Source: CAD feature listing. Evaluate the final solid. Frame: model axes, mm. Give positions to 0.01 mm unless a question says otherwise; leave off trailing zeros. Order: outer loops, then holes, each group sorted by start corner. A loop starts at its lowest first (then second) coordinate and runs counter-clockwise, first axis right, second up. Notation, with made-up numbers: M -7,-32.5 L 25,-32.5 A18 ccw 25,-8.5 Z; hole C -30,4.25 d1. An arc over 180 degrees is marked long. Use CSV: the item, a comma, the result in double quotes. Start each with the question number.
1. Line query: line 1 along Y through (x, z) = (-74, 1.45); line 2 along Y through (x, z) = (-49.5, 0.8); line 3 along X through (y, z) = (42, 2.15). Output: solid intervals per line, ascending. Write a range as [from, to].
2. Section query B-B, the plane y = 65. Return the cut outline in (x, z), plus the area to 3 significant figures.
3. Section query A-A, the plane x = -74. Return the cut outline in (y, z), plus the area to 3 significant figures.
4. Section query C-C, the plane z = 1.8. Return the cut outline in (x, y), plus the area to 3 significant figures.
from build123d import *

# Parameters (mm, degrees)
ESQUISSE1_W             = 152
ESQUISSE1_H             = 165
BOSS_EXTRU_1_DEPTH      = 3
CONG_1_R                = 5
ESQUISSE2_R             = 47.5
ENL_V_MAT_EXTRU_1_DEPTH = 3
ENL_V_MAT_EXTRU_2_DEPTH = 3


with BuildPart() as part:
    # Esquisse1 → Boss.-Extru.1 (new body)
    with BuildSketch(Plane.XY):
        with Locations((-76, 82.5)):
            Rectangle(ESQUISSE1_W, ESQUISSE1_H)
    extrude(amount=BOSS_EXTRU_1_DEPTH)

    # Congé1
    cong_1_edges = [part.edges().sort_by_distance(p)[0] for p in [
        (0, 0, 1.5),
        (-152, 0, 1.5),
        (-152, 165, 1.5),
        (0, 165, 1.5),
    ]]
    fillet(cong_1_edges, radius=CONG_1_R)

    # Esquisse2 → Enlèv. mat.-Extru.1 (cut)
    with BuildSketch(Plane(origin=(0, 0, 0), x_dir=(-1, 0, 0), z_dir=(0, 0, -1))):
        with Locations((74, 65)):
            Circle(ESQUISSE2_R)
    extrude(amount=-ENL_V_MAT_EXTRU_1_DEPTH, mode=Mode.SUBTRACT)

    # Esquisse3 → Enlèv. mat.-Extru.2 (cut)
    with BuildSketch(Plane(origin=(0, 0, 0), x_dir=(-1, 0, 0), z_dir=(0, 0, -1))):
        with BuildLine():
            Line((37, -3), (37, 3))
            ThreePointArc((37, 3), (41, 7), (45, 3))
            Line((45, 3), (45, -3))
            ThreePointArc((45, -3), (41, -7), (37, -3))
        make_face()
        with BuildLine():
            Line((103, -3), (103, 3))
            ThreePointArc((103, 3), (107, 7), (111, 3))
            Line((111, 3), (111, -3))
            ThreePointArc((111, -3), (107, -7), (103, -3))
        make_face()
    extrude(amount=-ENL_V_MAT_EXTRU_2_DEPTH, mode=Mode.SUBTRACT)


solid = part.part
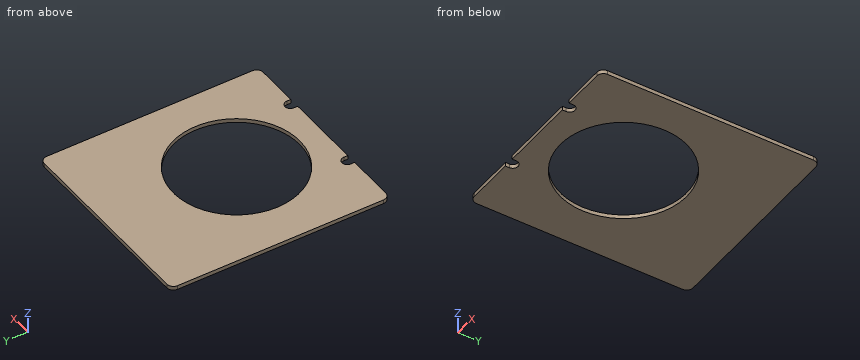
Result set:
1,line 1,"[0, 17.5], [112.5, 165]"
1,line 2,"[0, 24.31], [105.69, 165]"
1,line 3,"[-152, -115.56], [-32.44, 0]"
2,outline,"M -152,0 L -121.5,0 L -121.5,3 L -152,3 Z; M -26.5,0 L 0,0 L 0,3 L -26.5,3 Z"
2,area,"171 mm2"
3,outline,"M 0,0 L 17.5,0 L 17.5,3 L 0,3 Z; M 112.5,0 L 165,0 L 165,3 L 112.5,3 Z"
3,area,"210 mm2"
4,outline,"M -152,5 A5 ccw -147,0 L -111,0 L -111,3 A4 cw -103,3 L -103,0 L -45,0 L -45,3 A4 cw -37,3 L -37,0 L -5,0 A5 ccw 0,5 L 0,160 A5 ccw -5,165 L -147,165 A5 ccw -152,160 Z; hole C -74,65 d95"
4,area,"17,900 mm2"
